Can you work these out from the model? Positions are in its coordinate system, mm. A direction names the side the tool comes from. Coordinates: 2 decimals unless noted, no trailing zeros. Loops run counter-clockwise (first coordinate to the right, second up) from the corner with the lowest first, then second, coordinate; pieces in that order, holes last. Notation, with made-up numbers: (-31, 55) -> (-16, 55) arc R14 cw to (-16, 62) -> close; hole circle Ø4 at (34, 75). An arc over 180 degrees is marked (long way). Put each result on its own line as item: value. Start each with the question number.
Item 1: We'd pull the mould along Z, two halves only. Please class faces 1 (the flat face through (-6.005, 0.64, -11.4)), 2 (the cylindrical face through (-0.89, 0.64, 4.92)), 3 (the flat face through (-1, -15.9, 5)): pulls with the +Z half, pulls with the -Z half, needs draft (parallel to the pull), parting line crosses it, or undercut.
Item 2: If we section it at B-B on z = 11.5: Please give me the cut outline in (x, y), plus the area to 3 significant figures.
Item 3: If we section it at A-A on x = -12: Please give me the cut outline in (y, z), plus the area to 3 significant figures.
Item 4: If we section it at D-D on z = -15.5: Please give me the cut outline in (x, y).
Item 5: If we section it at C-C on x = -7: Please give me the cut outline in (y, z), plus the area to 3 significant figures.
Item 6: For faces 4 (the flat face through (-1, -17.75, 5)), 5 (the cylindrical face through (-3.905, 9.021, -0.867)), 6 (the cylindrical face through (-0.851, 0.64, -4.927)), 7 (the flat face through (-11.928, 0.64, 4.873)), 8 (the flat face through (-12.27, 0.64, 3.934)), which set-ups out of +Z, -Z, +X, -X, +Y, -Y let a thin tool reach every point of the face, with its end or its side?
Item 7: Will these pins go through, and if not, where does the flat tip stop? P1, Ø13, axis at x = 12, y = 2.5, coming from the +Z side; P2, Ø7, axis at x = 0, z = 0, coming from the +Y side; P3, Ø1.5, axis at x = 8, y = -1.5, coming from the +Z side.
Item 8: Please list where these lines run through material, in increasing order: L1, parallel to X at y = -17.05, z = 0; L2, parallel to X at y = -5, z = -8.5; L3, parallel to Z at x = 14, y = 1. Write a range as from..to.
```python
from build123d import *

# Parameters (mm, degrees)
SKETCH1_R           = 5
SKETCH1_R_2         = 3
BOSS_EXTRUDE2_DEPTH = 17.5
SKETCH4_W           = 18
SKETCH4_H           = 1
EXTRUDE_THIN1_DEPTH = 35
CIRPATTERN1_COUNT   = 9
SKETCH5_R           = 3
BOSS_EXTRUDE3_DEPTH = 15
SKETCH6_R           = 3.5
SKETCH6_R_2         = 1.5
CUT_EXTRUDE1_DEPTH  = 6
SKETCH15_R          = 1.5
CUT_EXTRUDE2_DEPTH  = 2
SKETCH17_R          = 2.5
BOSS_EXTRUDE4_DEPTH = 3
SKETCH18_R          = 2
CUT_EXTRUDE3_DEPTH  = 2
SKETCH19_R          = 4
CUT_EXTRUDE4_DEPTH  = 20
SKETCH20_W          = 45.677284088
SKETCH20_H          = 45.724664858
CUT_EXTRUDE5_DEPTH  = 8
SKETCH21_R          = 3
BOSS_EXTRUDE5_DEPTH = 1
SKETCH24_R          = 9.912143672
BOSS_EXTRUDE6_DEPTH = 0.5
SKETCH25_R          = 3.2
CUT_EXTRUDE6_DEPTH  = 2.1
SKETCH26_R          = 3.2
BOSS_EXTRUDE7_DEPTH = 0.25
CUT_EXTRUDE8_START  = -7.5
CUT_EXTRUDE8_DEPTH  = 7.5
SKETCH28_R          = 0.5
CUT_EXTRUDE9_DEPTH  = 1.5
CUT_EXTRUDE10_DEPTH = 7
BOSS_EXTRUDE8_START = 10
SKETCH30_R          = 4
BOSS_EXTRUDE8_DEPTH = 10


with BuildPart() as part:
    # Sketch1 → Boss-Extrude2 (new, symmetric)
    with BuildSketch(Plane(origin=(0, 0, 0), x_dir=(1, 0, 0), z_dir=(0, 1, 0))):
        with Locations(Location((0, 0, 0), (0, 0, 270))):
            Circle(SKETCH1_R)
        with Locations(Location((0, 0, 0), (0, 0, 270))):
            Circle(SKETCH1_R_2, mode=Mode.SUBTRACT)
    extrude(amount=BOSS_EXTRUDE2_DEPTH, both=True)

    # Sketch4 → Extrude-Thin1 (add)
    with BuildSketch(Plane(origin=(0, 17.5, 0), x_dir=(1, 0, 0), z_dir=(0, 1, 0))):
        with Locations((12, 0)):
            Rectangle(SKETCH4_W, SKETCH4_H)
    extrude_thin1 = extrude(amount=-EXTRUDE_THIN1_DEPTH)

    # CirPattern1: Extrude-Thin1 ×9 about axis
    cirpattern1_axis = Axis((0, 0, 0), (0, 1, 0))
    for i in range(1, CIRPATTERN1_COUNT):
        add(extrude_thin1.rotate(cirpattern1_axis, i * 360 / CIRPATTERN1_COUNT))

    # Sketch5 → Boss-Extrude3 (add)
    with BuildSketch(Plane(origin=(0, -17.5, 0), x_dir=(-1, 0, 0), z_dir=(0, -1, 0))):
        with Locations(Location((0, 0, 0), (0, 0, 90))):
            Circle(SKETCH5_R)
    extrude(amount=-BOSS_EXTRUDE3_DEPTH)

    # Sketch6 → Cut-Extrude1 (cut)
    with BuildSketch(Plane(origin=(0, -17.5, 0), x_dir=(-1, 0, 0), z_dir=(0, -1, 0))):
        with Locations(Location((0, 0, 0), (0, 0, 90))):
            Circle(SKETCH6_R)
        with Locations(Location((0, 0, 0), (0, 0, 90))):
            Circle(SKETCH6_R_2, mode=Mode.SUBTRACT)
    extrude(amount=-CUT_EXTRUDE1_DEPTH, mode=Mode.SUBTRACT)

    # Sketch15 → Cut-Extrude2 (cut)
    with BuildSketch(Plane.XZ.offset(17.5)):
        with Locations(Location((0, 0, 0), (0, 0, 270))):
            Circle(SKETCH15_R)
    extrude(amount=-CUT_EXTRUDE2_DEPTH, mode=Mode.SUBTRACT)

    # Sketch17 → Boss-Extrude4 (add)
    with BuildSketch(Plane.XZ.offset(17.5)):
        with Locations((18.5, 0)):
            Circle(SKETCH17_R)
    extrude(amount=-BOSS_EXTRUDE4_DEPTH)

    # Sketch18 → Cut-Extrude3 (cut)
    with BuildSketch(Plane.XZ.offset(17.5)):
        with Locations(Location((18.5, 0, 0), (0, 0, 270))):
            Circle(SKETCH18_R)
    extrude(amount=-CUT_EXTRUDE3_DEPTH, mode=Mode.SUBTRACT)

    # Sketch19 → Cut-Extrude4 (cut)
    with BuildSketch(Plane(origin=(0, 17.5, 0), x_dir=(1, 0, 0), z_dir=(0, 1, 0))):
        with Locations(Location((0, 0, 0), (0, 0, 270))):
            Circle(SKETCH19_R)
    extrude(amount=-CUT_EXTRUDE4_DEPTH, mode=Mode.SUBTRACT)

    # Sketch20 → Cut-Extrude5 (cut)
    with BuildSketch(Plane(origin=(0, -17.5, 0), x_dir=(-1, 0, 0), z_dir=(0, -1, 0))):
        Rectangle(SKETCH20_W, SKETCH20_H)
    extrude(amount=-CUT_EXTRUDE5_DEPTH, mode=Mode.SUBTRACT)

    # Sketch21 → Boss-Extrude5 (add)
    with BuildSketch(Plane.XZ.offset(9.5)):
        with Locations(Location((0, 0, 0), (0, 0, 90))):
            Circle(SKETCH21_R)
    extrude(amount=BOSS_EXTRUDE5_DEPTH)

    # Sketch23 → Revolve1 (revolve)
    with BuildSketch(Plane(origin=(0, 0, 0), x_dir=(0, 0, -1), z_dir=(1, 0, 0))):
        with BuildLine():
            Line((-3, -10.5), (-2, -10.5))
            Line((-2, -10.5), (0, -10.5))
            Line((0, -10.5), (0, -17.5))
            Line((0, -17.5), (-8.912143672, -17.5))
            Line((-8.912143672, -17.5), (-9.912143672, -17.5))
            ThreePointArc((-9.912143672, -17.5), (-7.260403323, -13.2057636), (-3, -10.5))
        make_face()
    revolve(axis=Axis((0, -11.130650603, 0), (0, -1, 0)))

    # Sketch24 → Boss-Extrude6 (add)
    with BuildSketch(Plane.XZ.offset(17.5)):
        with Locations(Location((0, 0, 0), (0, 0, 270))):
            Circle(SKETCH24_R)
    extrude(amount=BOSS_EXTRUDE6_DEPTH)

    # Sketch25 → Cut-Extrude6 (cut)
    with BuildSketch(Plane.XZ.offset(18)):
        with Locations(Location((-0.56668442, 5, 0), (0, 0, 270))):
            Circle(SKETCH25_R)
    extrude(amount=-CUT_EXTRUDE6_DEPTH, mode=Mode.SUBTRACT)

    # Sketch26 → Boss-Extrude7 (add)
    with BuildSketch(Plane.XZ.offset(18)):
        with Locations(Location((-0.56668442, 5, 0), (0, 0, 270))):
            Circle(SKETCH26_R)
    extrude(amount=-BOSS_EXTRUDE7_DEPTH)

    # Sketch27 → Cut-Extrude8 (cut)
    with BuildSketch(Plane.XZ.offset(18).offset(CUT_EXTRUDE8_START)):
        with BuildLine():
            ThreePointArc((-5.368630905, 4.991892601), (-6.424807204, 5.779358473), (-7.613826501, 6.346671425))
            ThreePointArc((-7.613826501, 6.346671425), (-9.912143672, 0), (-7.613826501, -6.346671425))
            ThreePointArc((-7.613826501, -6.346671425), (-6.424807204, -5.779358473), (-5.368630905, -4.991892601))
            ThreePointArc((-5.368630905, -4.991892601), (-3.162143672, 0), (-5.368630905, 4.991892601))
        make_face()
        with BuildLine():
            ThreePointArc((9.912143672, 0), (9.319869483, 3.375), (7.613826501, 6.346671425))
            ThreePointArc((7.613826501, 6.346671425), (6.424807204, 5.779358473), (5.368630905, 4.991892601))
            ThreePointArc((5.368630905, 4.991892601), (3.162143672, 0), (5.368630905, -4.991892601))
            ThreePointArc((5.368630905, -4.991892601), (6.424807204, -5.779358473), (7.613826501, -6.346671425))
            ThreePointArc((7.613826501, -6.346671425), (9.319869483, -3.375), (9.912143672, 0))
        make_face()
        with BuildLine():
            ThreePointArc((-5.368630905, -4.991892601), (-6.424807204, -5.779358473), (-7.613826501, -6.346671425))
            ThreePointArc((-7.613826501, -6.346671425), (-4.203657524, -8.976628297), (0, -9.912143672))
            add(Edge.make_bspline(
                [(-5.368630905, -4.991892601), (-4.998119196, -7.539682857), (-2.616364035, -9.837937814), (0, -9.912143672)],
                knots=[0, 0, 0, 0, 1, 1, 1, 1], degree=3))
        make_face()
        with BuildLine():
            add(Edge.make_bspline(
                [(5.368630905, -4.991892601), (4.998119196, -7.539682857), (2.616364035, -9.837937814), (0, -9.912143672)],
                knots=[0, 0, 0, 0, 1, 1, 1, 1], degree=3))
            ThreePointArc((0, -9.912143672), (4.203657524, -8.976628297), (7.613826501, -6.346671425))
            ThreePointArc((7.613826501, -6.346671425), (6.424807204, -5.779358473), (5.368630905, -4.991892601))
        make_face()
        with BuildLine():
            ThreePointArc((0, 9.912143672), (-4.203657524, 8.976628297), (-7.613826501, 6.346671425))
            ThreePointArc((-7.613826501, 6.346671425), (-6.424807204, 5.779358473), (-5.368630905, 4.991892601))
            add(Edge.make_bspline(
                [(-5.368630905, 4.991892601), (-4.998119196, 7.539682857), (-2.616364035, 9.837937814), (0, 9.912143672)],
                knots=[0, 0, 0, 0, 1, 1, 1, 1], degree=3))
        make_face()
        with BuildLine():
            ThreePointArc((7.613826501, 6.346671425), (4.203657524, 8.976628297), (0, 9.912143672))
            add(Edge.make_bspline(
                [(5.368630905, 4.991892601), (4.998119196, 7.539682857), (2.616364035, 9.837937814), (0, 9.912143672)],
                knots=[0, 0, 0, 0, 1, 1, 1, 1], degree=3))
            ThreePointArc((5.368630905, 4.991892601), (6.424807204, 5.779358473), (7.613826501, 6.346671425))
        make_face()
    extrude(amount=CUT_EXTRUDE8_DEPTH, mode=Mode.SUBTRACT)

    # Sketch28 → Cut-Extrude9 (cut)
    with BuildSketch(Plane.XZ.offset(18)):
        with Locations(Location((0, 0, 0), (0, 0, 270))):
            Circle(SKETCH28_R)
    extrude(amount=-CUT_EXTRUDE9_DEPTH, mode=Mode.SUBTRACT)

    # Sketch29 → Cut-Extrude10 (cut)
    with BuildSketch(Plane(origin=(0, 17.5, 0), x_dir=(1, 0, 0), z_dir=(0, 1, 0))):
        with BuildLine():
            Line((3.489629181, -3.580850203), (15.765539501, -13.881562025))
            Line((15.765539501, -13.881562025), (16.40832711, -13.115517582))
            Line((16.40832711, -13.115517582), (4.132416791, -2.81480576))
            ThreePointArc((4.132416791, -2.81480576), (4.698463104, -1.710100717), (4.974937186, -0.5))
            Line((4.974937186, -0.5), (21, -0.5))
            Line((21, -0.5), (21, 0.5))
            Line((21, 0.5), (4.974937186, 0.5))
            ThreePointArc((4.974937186, 0.5), (4.698463104, 1.710100717), (4.132416791, 2.81480576))
            Line((4.132416791, 2.81480576), (16.40832711, 13.115517582))
            Line((16.40832711, 13.115517582), (15.765539501, 13.881562025))
            Line((15.765539501, 13.881562025), (3.489629181, 3.580850203))
            ThreePointArc((3.489629181, 3.580850203), (2.5, 4.330127019), (1.356292653, 4.812532622))
            Line((1.356292653, 4.812532622), (4.139015608, 20.594138724))
            Line((4.139015608, 20.594138724), (3.154207854, 20.767786902))
            Line((3.154207854, 20.767786902), (0.3714849, 4.9861808))
            ThreePointArc((0.3714849, 4.9861808), (-0.868240888, 4.924038765), (-2.054455891, 4.558421985))
            Line((-2.054455891, 4.558421985), (-10.066987298, 18.436533479))
            Line((-10.066987298, 18.436533479), (-10.933012702, 17.936533479))
            Line((-10.933012702, 17.936533479), (-2.920481295, 4.058421985))
            ThreePointArc((-2.920481295, 4.058421985), (-3.830222216, 3.213938048), (-4.50390169, 2.17137504))
            Line((-4.50390169, 2.17137504), (-19.562534965, 7.65226932))
            Line((-19.562534965, 7.65226932), (-19.904555108, 6.712576699))
            Line((-19.904555108, 6.712576699), (-4.845921834, 1.231682419))
            ThreePointArc((-4.845921834, 1.231682419), (-5, 0), (-4.845921834, -1.231682419))
            Line((-4.845921834, -1.231682419), (-19.904555108, -6.712576699))
            Line((-19.904555108, -6.712576699), (-19.562534965, -7.65226932))
            Line((-19.562534965, -7.65226932), (-4.50390169, -2.17137504))
            ThreePointArc((-4.50390169, -2.17137504), (-3.830222216, -3.213938048), (-2.920481295, -4.058421985))
            Line((-2.920481295, -4.058421985), (-10.933012702, -17.936533479))
            Line((-10.933012702, -17.936533479), (-10.066987298, -18.436533479))
            Line((-10.066987298, -18.436533479), (-2.054455891, -4.558421985))
            ThreePointArc((-2.054455891, -4.558421985), (-0.868240888, -4.924038765), (0.3714849, -4.9861808))
            Line((0.3714849, -4.9861808), (3.154207854, -20.767786902))
            Line((3.154207854, -20.767786902), (4.139015608, -20.594138724))
            Line((4.139015608, -20.594138724), (1.356292653, -4.812532622))
            ThreePointArc((1.356292653, -4.812532622), (2.5, -4.330127019), (3.489629181, -3.580850203))
        make_face()
    extrude(amount=-CUT_EXTRUDE10_DEPTH, mode=Mode.SUBTRACT)

    # Sketch30 → Boss-Extrude8 (add)
    with BuildSketch(Plane(origin=(0, -2.5, 0), x_dir=(1, 0, 0), z_dir=(0, 1, 0)).offset(BOSS_EXTRUDE8_START)):
        with Locations(Location((0, 0, 0), (0, 0, 270))):
            Circle(SKETCH30_R)
    extrude(amount=-BOSS_EXTRUDE8_DEPTH)


solid = part.part
```
Solutions:
1. face 1: pulls with the -Z half
1. face 2: pulls with the +Z half
1. face 3: undercut
2. outline: (-7.22, -9.5) -> (-6.06, -9.5) -> (-6.06, 10.5) -> (-7.22, 10.5) -> close; (1.52, -9.5) -> (2.54, -9.5) -> (2.54, 10.5) -> (1.52, 10.5) -> close; (12.93, -9.5) -> (14.48, -9.5) -> (14.48, 10.5) -> (12.93, 10.5) -> close
2. area: 74.5 mm^2
3. outline: (-9.5, -4.9) -> (10.5, -4.9) -> (10.5, -3.84) -> (-9.5, -3.84) -> close; (-9.5, 3.84) -> (10.5, 3.84) -> (10.5, 4.9) -> (-9.5, 4.9) -> close
3. area: 42.6 mm^2
4. outline: (-9.53, -9.5) -> (-8.37, -9.5) -> (-8.37, 10.5) -> (-9.53, 10.5) -> close; (2.23, -9.5) -> (3.24, -9.5) -> (3.24, 10.5) -> (2.23, 10.5) -> close
5. outline: (-9.5, -13.12) -> (10.5, -13.12) -> (10.5, -11.12) -> (-9.5, -11.12) -> close; (-9.5, -3.08) -> (10.5, -3.08) -> (10.5, -2.02) -> (-9.5, -2.02) -> close; (-9.5, 2.02) -> (10.5, 2.02) -> (10.5, 3.08) -> (-9.5, 3.08) -> close; (-9.5, 11.12) -> (10.5, 11.12) -> (10.5, 13.12) -> (-9.5, 13.12) -> close
5. area: 123 mm^2
6. face 4: none
6. face 5: +Y
6. face 6: -Z, +Y
6. face 7: +Y, -Y
6. face 8: -X, +Y, -Y
7. P1: z = 13.88
7. P2: y = 7.5
7. P3: z = 7.99
8. L1: -3.16..-0.5, 0.5..3.16
8. L2: -5.48..-4.33, 0.99..2.01, 9.35..10.91
8. L3: -12.4..-11.09, -0.5..0.5, 11.09..12.4
